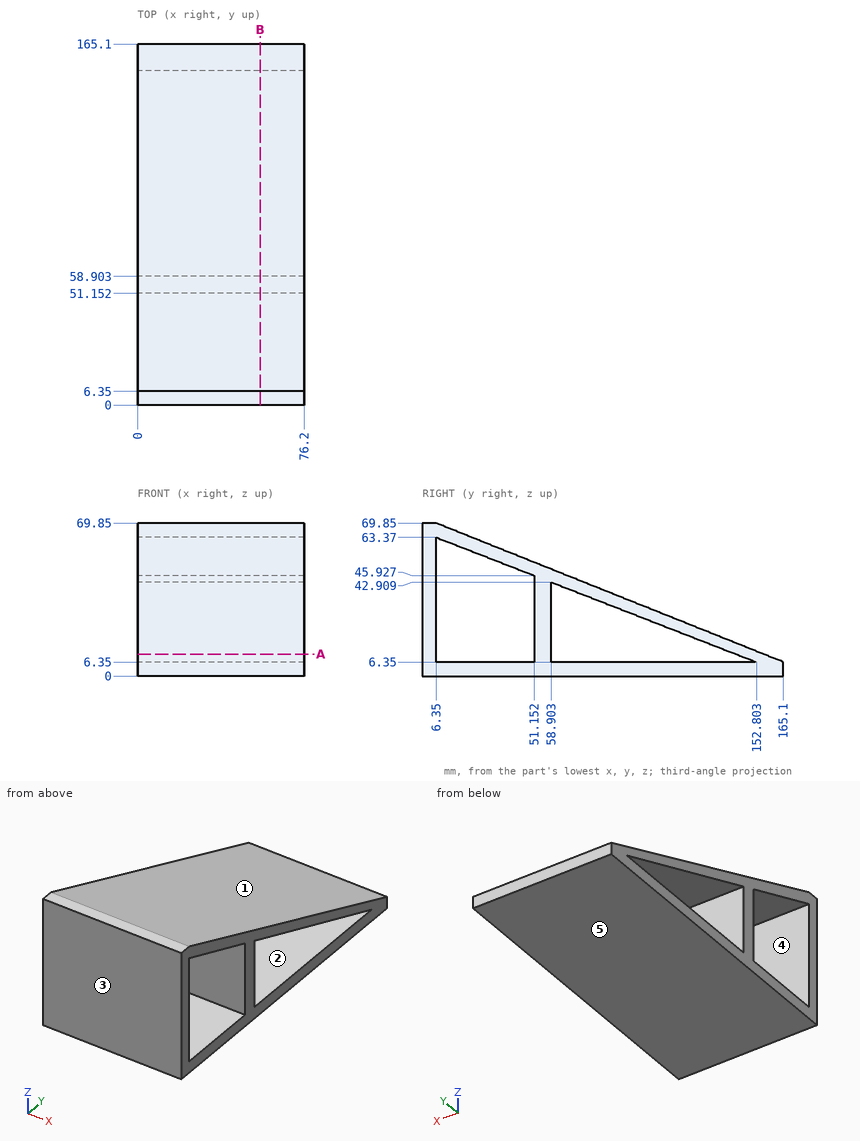
Study the drawing (mm; zero at the part's minimum x, y, z) and answer. A direction names the side the tool comes from. Round coordinates to 2 decimals unless told otherwise and drop trailing zeros. Write each loop counter-clockwise with the first axis right and the second up, starting at its lowest first coordinate (ties: lowest second). Pieces come first, ordered by that corner, then holes.
Q1. A tool of negligible diameter and unlimited length cuts with its end or side. For the marked faces 1 and 2, from which of +Z, -Z, +X, -X, +Y, -Y can it reach the whole face along a straight path? Write none if from no direction.
Values:
face 1: +Z, +X, -X, +Y
face 2: +X, -X
Q2. Find section A-A on z = 10. State how many separate pieces and enclosed holes the cut face has, and give its area (3 significant figures).
Values:
separate pieces: 3
enclosed holes: 0
area: 2,030 mm2
Q3. Find section B-B on x = 56. Determine the outline of the cut face in (y, z), and give its area (3 significant figures).
Values:
outline: (0, 0) - (165.1, 0) - (165.1, 6.35) - (6.35, 69.85) - (0, 69.85) - close; hole (6.35, 6.35) - (51.15, 6.35) - (51.15, 45.93) - (6.35, 63.37) - close; hole (58.9, 6.35) - (152.8, 6.35) - (58.9, 42.91) - close
area: 2,610 mm2
Q4. The mould has two halves that part along Z. Classify the marked faces 3, 4 and 5: released by +Z, released by -Z, zero draft, split by the parting line, or undercut.
Values:
face 3: zero draft
face 4: undercut
face 5: released by -Z
Q5. Straight lines are drawn through the part: line 1 (Z direction, x = 29, y = 60); line 2 (Z direction, x = 43.5, y = 140.5). For each, find the intervals that lie inside material, in ascending order.
Values:
line 1: z = 0 to 6.35, 42.48 to 48.39
line 2: z = 0 to 6.35, 11.14 to 16.19
Q6. Flat-ended cylindrical pins translate along their axes: P1, Ø20, axis at x = 25, z = 21, coming from the -Y side; P2, Ø4, axis at x = 9, y = 65, coming from the +Z side; P3, Ø23, axis at x = 52.5, y = 116, coming from the +Z side; P4, Ø5, axis at x = 13, y = 57, coming from the +Z side. Find the tip coordinate at first contact, or state that the pin passes through.
Values:
P1: stops at y = 0
P2: stops at z = 47.19
P3: stops at z = 30.59
P4: stops at z = 50.59
